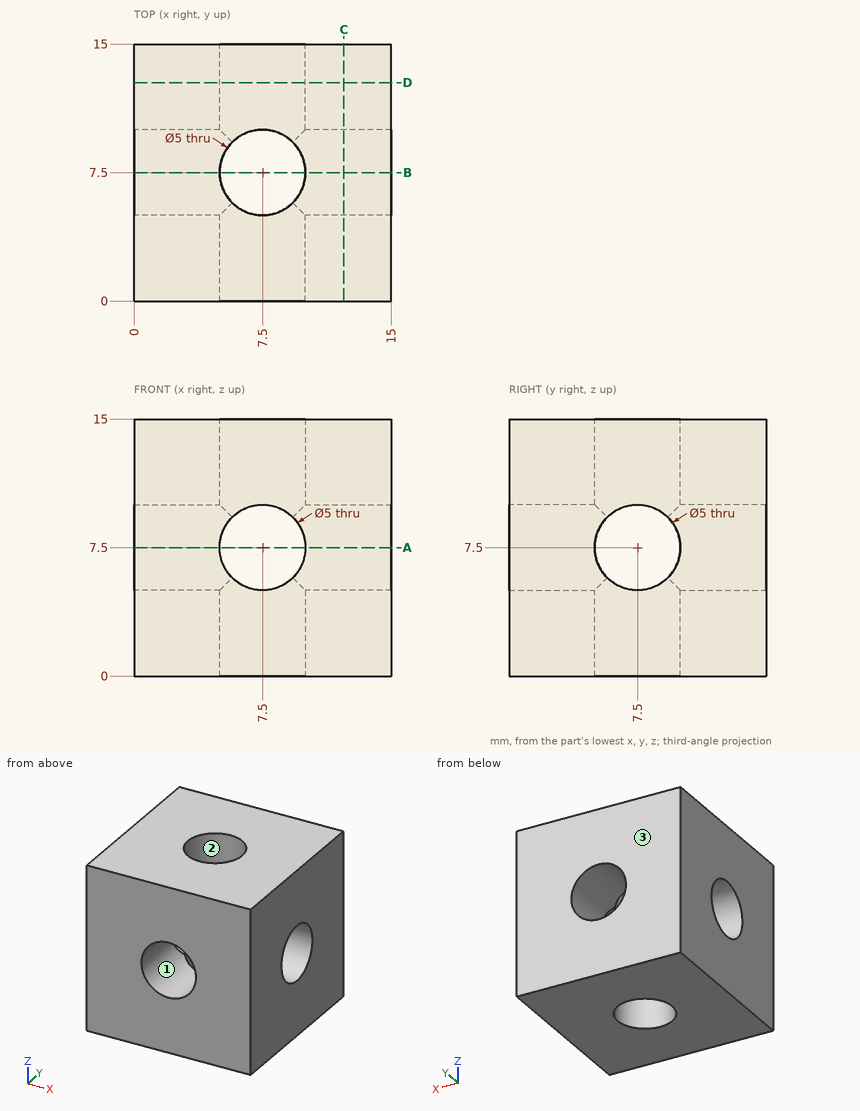
Can you work these out from the drawing? Everything is in mm from the part's minimum corner. Coordinates: 2 decimals unless noted, no trailing zeros. Loops run counter-clockwise (first coordinate to the right, second up) from the corner with the lowest first, then second, coordinate; pieces in that order, holes last.
1) Imagine slicing it at C-C on x = 12.25. List the corners of the cut face in (y, z) for me.
2) Thinking about a two-plate mould opening in Y: for the marked faces 1, 2 and 3, which applies, pulls with the +Y half, pulls with the -Y half, needs draft (parallel to the pull), parting line crosses it, or undercut?
3) I need wall thicknesses on probe 1 along Y at (x, z) = (7.5, 10.9). Which ranges of the line are inside material? Lowest first, please.
4) Imagine slicing it at A-A on z = 7.5. List the corners of the cut face in (x, y) for me.
5) For pin 1 (3 mm diameter, centred on x = 7.5, y = 7.5, fed in from +Z), with a flat end and sliding along its axis, tell me the tip position at first contact or that it passes through.
Completed:
1. outline: (0, 0) - (15, 0) - (15, 15) - (0, 15) - close; hole circle Ø5 at (7.5, 7.5)
2. face 1: needs draft
2. face 2: undercut
2. face 3: pulls with the +Y half
3. probe 1: y = 0 to 5, 10 to 15
4. outline: (0, 0) - (5, 0) - (5, 5) - (0, 5) - close; (0, 10) - (5, 10) - (5, 15) - (0, 15) - close; (10, 0) - (15, 0) - (15, 5) - (10, 5) - close; (10, 10) - (15, 10) - (15, 15) - (10, 15) - close
5. pin 1: passes through
